Design review of the part built by this model. Coordinates are the model's own, in mm. Face numbers are marked on the shaded views. A direction names the side the tool comes from. Round coordinates to 2 decimals unless told otherwise and drop trailing zeros. Order: outer loops, then holes, each group sorted by start corner. A loop starts at its lowest first (then second) coordinate and runs counter-clockwise, first axis right, second up. Notation, with made-up numbers: M 79.5,21 L 93.5,21 A16 ccw 93.5,47 Z; hole C 61,52 d4. An arc over 180 degrees is marked long. Use a Markdown table: item, result. Add a question column.
(1) Machinability: for the marked faces 1 and 2, which of the approach directions +Z, -Z, +X, -X, +Y, -Y give a long, thin tool a straight path to every point of the face, cutting with its end or side? Answer none if there is none.
(2) Take a section at C-C (x = 0.5). Write out the cut boundary in (y, z).
(3) The part is to be moulded in two halves that separate along Z. For the marked faces 3, 4 and 5, say which applies: released by +Z, released by -Z, zero draft, split by the parting line, or undercut.
(4) For pin 1 (0.6 mm diameter, centred on y = 5, z = -2, fed in from +X); pin 2 (2 mm diameter, centred on x = -5.5, z = -4, fed in from +Y), all flat-tipped, find the tip position at first contact; note any pin that passes through.
(5) Take a section at B-B (y = 3). Write out the cut boundary in (x, z).
(6) Take a section at D-D (z = 3.5). Write out the cut boundary in (x, y), then the cut area to 3 significant figures.
(7) To check wall thickness, follow probe 1 along Z at (x, y) = (0, 2); probe 2 along X at (y, z) = (4.5, 0). State the ranges of each line that lie inside material, in increasing order. Write a range as from..to.
(8) Take a section at A-A (z = 0). Write out the cut boundary in (x, y), then the cut area to 3 significant figures.
```python
from build123d import *

# Parameters (mm, degrees)
BOSS_EXTRUDE1_DEPTH      = 8
BOSS_EXTRUDE1_DEPTH_BACK = 8
SKETCH9_R                = 3
CUT_EXTRUDE2_DEPTH       = 7
FILLET1_R                = 0.3


with BuildPart() as part:
    # Sketch4 → Boss-Extrude1 (new body, two sides)
    with BuildSketch(Plane.XY) as boss_extrude1_sk:
        Polygon((-8, 4.2), (-8, 2.5), (-5.5, 0), (5.5, 0), (8, 2.5), (8, 4.2), (3.9, 4.2), (3.9, 6), (0.891031267, 6), (0, 5.64), (-0.891031267, 6), (-3.9, 6), (-3.9, 4.2), align=None)
    extrude(amount=BOSS_EXTRUDE1_DEPTH)
    extrude(boss_extrude1_sk.sketch, amount=-BOSS_EXTRUDE1_DEPTH_BACK)

    # Sketch9 → Cut-Extrude2 (cut, through all)
    with BuildSketch(Plane(origin=(0, 0, 0), x_dir=(1, 0, 0), z_dir=(0, 1, 0))):
        Circle(SKETCH9_R)
    extrude(amount=CUT_EXTRUDE2_DEPTH, mode=Mode.SUBTRACT)

    # Fillet1
    fillet1_edges = [part.edges().sort_by_distance(p)[0] for p in [
        (-3.9, 6, 0),
        (-3.9, 4.2, 0),
        (-8, 4.2, 0),
        (-8, 2.5, 0),
        (-5.5, 0, 0),
        (5.5, 0, 0),
        (8, 2.5, 0),
        (8, 4.2, 0),
        (3.9, 4.2, 0),
        (3.9, 6, 0),
        (0, 5.64, -5.5),
        (0, 5.64, 5.5),
    ]]
    fillet(fillet1_edges, radius=FILLET1_R)


solid = part.part
```
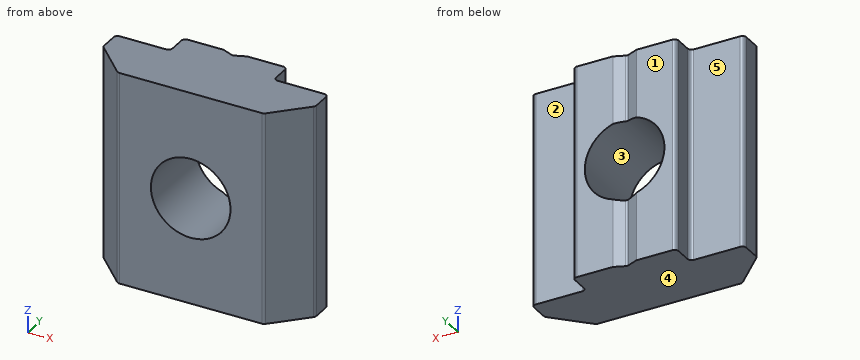
Verdict:
| question | item | result |
|---|---|---|
| 1 | face 1 | +Z, -Z, +X, -X, +Y |
| 1 | face 2 | +Z, -Z, +X, +Y |
| 2 | outline | M 0,-8 L 5.84,-8 L 5.84,-2.96 L 0,-2.96 Z; M 0,2.96 L 5.84,2.96 L 5.84,8 L 0,8 Z |
| 3 | face 3 | undercut |
| 3 | face 4 | released by -Z |
| 3 | face 5 | zero draft |
| 4 | pin 1 | stops at x = 3.9 |
| 4 | pin 2 | stops at y = 4.2 |
| 5 | outline | M -8,-8 L 8,-8 L 8,8 L -8,8 Z; hole C 0,0 d6 |
| 6 | outline | M -8,2.62 A0.3 ccw -7.91,2.41 L -5.59,0.09 A0.3 ccw -5.38,0 L 5.38,0 A0.3 ccw 5.59,0.09 L 7.91,2.41 A0.3 ccw 8,2.62 L 8,3.9 A0.3 ccw 7.7,4.2 L 4.2,4.2 A0.3 cw 3.9,4.5 L 3.9,5.7 A0.3 ccw 3.6,6 L 0.89,6 L 0.11,5.69 A0.3 cw -0.11,5.69 L -0.89,6 L -3.6,6 A0.3 ccw -3.9,5.7 L -3.9,4.5 A0.3 cw -4.2,4.2 L -7.7,4.2 A0.3 ccw -8,3.9 Z |
| 6 | area | 74.6 mm^2 |
| 7 | probe 1 | z = -8..-3, 3..8 |
| 7 | probe 2 | x = -3.9..-3, 3..3.9 |
| 8 | outline | M -8,2.62 A0.3 ccw -7.91,2.41 L -5.59,0.09 A0.3 ccw -5.38,0 L -3,0 L -3,6 L -3.6,6 A0.3 ccw -3.9,5.7 L -3.9,4.5 A0.3 cw -4.2,4.2 L -7.7,4.2 A0.3 ccw -8,3.9 Z; M 3,0 L 5.38,0 A0.3 ccw 5.59,0.09 L 7.91,2.41 A0.3 ccw 8,2.62 L 8,3.9 A0.3 ccw 7.7,4.2 L 4.2,4.2 A0.3 cw 3.9,4.5 L 3.9,5.7 A0.3 ccw 3.6,6 L 3,6 Z |
| 8 | area | 38.9 mm^2 |
